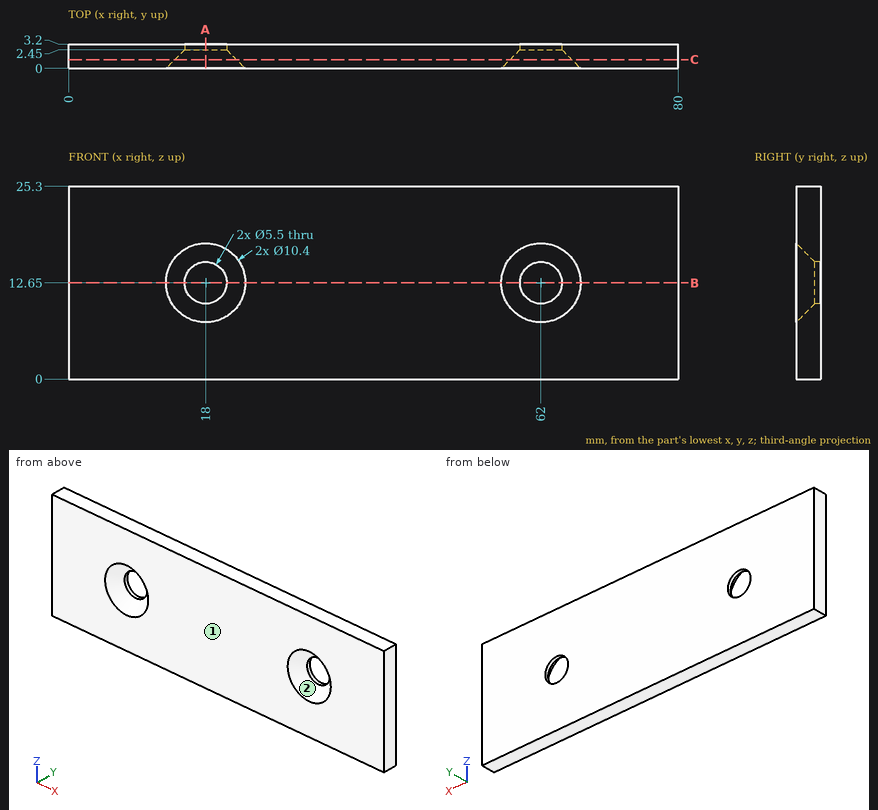
Print and shaded views of the part. All mm, measured from the part's lowest x, y and z. Round coordinates to 2 decimals unless told otherwise and drop trailing zeros. Order: outer loops, then holes, each group sorted by start corner. A loop starts at its lowest first (then second) coordinate and runs counter-clockwise, first axis right, second up.
Q1. Two-plate mould, pull along Z, no slides. Class the marked faces 1 and 2: pulls with the +Z half, pulls with the -Z half, needs draft (parallel to the pull), parting line crosses it, or undercut.
Q2. Wall check: L1, parallel to X at y = 2.7, z = 12.65; L2, parallel to Z at x = 62, y = 2.8; L3, parallel to X at y = 0.4, z = 16.25. Give the ranges that are in metal, low to high.
Q3. Slice it at B-B (z = 12.65). Write the cut outline in (x, y).
Q4. Drop a flat-ended pin along its axis: pin 1 (9 mm diameter, centred on x = 62, z = 12.65, fed in from +Y). Give the stop position or say it passes through.
Q5. Slice it at C-C (y = 1.15). Write the cut outline in (x, z).
Q6. Slice it at A-A (x = 18). Write the cut outline in (y, z), and give its area (3 significant figures).
Results below:
1. face 1: needs draft
1. face 2: undercut
2. L1: x = 0 to 15.25, 20.75 to 59.25, 64.75 to 80
2. L2: z = 0 to 9.9, 15.4 to 25.3
2. L3: x = 0 to 14.83, 21.17 to 58.83, 65.17 to 80
3. outline: (0, 0) - (12.8, 0) - (15.25, 2.45) - (15.25, 3.2) - (0, 3.2) - close; (20.75, 2.45) - (23.2, 0) - (56.8, 0) - (59.25, 2.45) - (59.25, 3.2) - (20.75, 3.2) - close; (64.75, 2.45) - (67.2, 0) - (80, 0) - (80, 3.2) - (64.75, 3.2) - close
4. pin 1: stops at y = 3.2
5. outline: (0, 0) - (80, 0) - (80, 25.3) - (0, 25.3) - close; hole circle Ø8.1 at (18, 12.65); hole circle Ø8.1 at (62, 12.65)
6. outline: (0, 0) - (3.2, 0) - (3.2, 9.9) - (2.45, 9.9) - (0, 7.45) - close; (0, 17.85) - (2.45, 15.4) - (3.2, 15.4) - (3.2, 25.3) - (0, 25.3) - close
6. area: 57.4 mm2
